CAD build for the part. Positions are in the model's coordinates, mm. Face numbers are marked on the shaded views. A direction names the side the tool comes from. Coordinates: 2 decimals unless noted, no trailing zeros. Order: outer loops, then holes, each group sorted by start corner. A loop starts at its lowest first (then second) coordinate and runs counter-clockwise, first axis right, second up. Notation, with made-up numbers: M -26,89 L -22,89 A21 cw -22,110 Z; hole C 58.5,19.5 d7. An arc over 180 degrees is marked long. Write item = value, one per line.
from build123d import *

# Parameters (mm, degrees)
F1_DEPTH = 60
F3_DEPTH = 2.001
F5_DEPTH = 1
F6_W     = 0.8
F6_H     = 3
F7_DEPTH = 1


# Not quite as in the source:
# - a feature names something its author has since deleted; it is built from what else it names


with BuildPart() as f1:
    # F0 (on Front) → F1 (new body)
    with BuildSketch(Plane.XZ):
        Polygon((0, 10), (0, 0), (16, 0), (16, 6), (13, 6.75), (13, 2), (3, 2), (3, 9.25), align=None)
    extrude(amount=F1_DEPTH)

    # F2 (on face) → F3 (cut, through all)
    with BuildSketch(Plane.XY.offset(2)):
        with BuildLine():
            ThreePointArc((12, -20.5), (8, -16.5), (4, -20.5))
            Line((4, -20.5), (4, -39.5))
            ThreePointArc((4, -39.5), (8, -43.5), (12, -39.5))
            Line((12, -39.5), (12, -20.5))
        make_face()
    extrude(amount=-F3_DEPTH, mode=Mode.SUBTRACT)

    # F4 (on Top) → F5 (cut)
    with BuildSketch(Plane.XY):
        with BuildLine():
            ThreePointArc((13, -20.5), (8, -15.5), (3, -20.5))
            Line((3, -20.5), (3, -39.5))
            ThreePointArc((3, -39.5), (8, -44.5), (13, -39.5))
            Line((13, -39.5), (13, -20.5))
        make_face()
    extrude(amount=F5_DEPTH, mode=Mode.SUBTRACT)

    # F6 (on Top) → F7 (join)
    with BuildSketch(Plane.XY):
        with Locations((6.8, -4.5)):
            Rectangle(F6_W, F6_H)
        with Locations((6.8, -55.5)):
            Rectangle(F6_W, F6_H)
    extrude(amount=-F7_DEPTH)


solid = f1.part
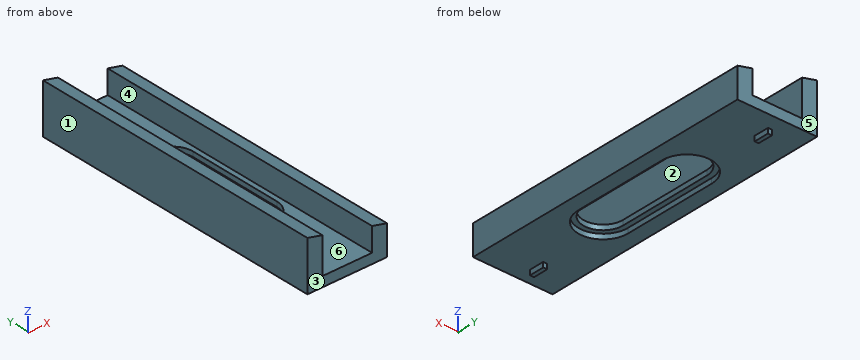
(1) Slice it at D-D, the plane y = -50. Write the cut outline in (x, z).
Evaluation:
outline = M 0,0 L 16,0 L 16,6 L 13,6.75 L 13,2 L 3,2 L 3,9.25 L 0,10 Z
(2) Pin check, flat tips, straight feed: pin 1 Ø5 at (x, y) = (6, -24.5) entering from -Z; pin 2 Ø5 at (x, y) = (12.5, -14) entering from +Z; pin 3 Ø0.5 at (y, z) = (-4.5, -0.5) entering from +X; pin 4 Ø3 at (x, y) = (9, -27) entering from -Z. Stop position of each tip, or through.
Evaluation:
pin_1 = 1
pin_2 = 6.75
pin_3 = 7.2
pin_4 = through
(3) Tool access for the marked faces 5 and 6: list every direction of +Z, -Z, +X, -X, +Y, -Y with a clear straight run to the whole face (end or side of a thin tool).
Evaluation:
face_5 = +Z, -Z, +X, -X, +Y
face_6 = +Z, +Y, -Y
(4) Pull direction X, two halves, no side cores. Call the marked faces 1, 2, 3 and 4: +X half, -X half, draft (parallel to the pull), parting line (faces both ways), or undercut.
Evaluation:
face_1 = -X half
face_2 = undercut
face_3 = draft
face_4 = undercut
(5) Slice it at C-C, the plane x = 8. Write the cut outline in (y, z).
Evaluation:
outline = M -60,0 L -44.5,0 L -44.5,1 L -43.5,1 L -43.5,2 L -60,2 Z; M -16.5,1 L -15.5,1 L -15.5,0 L 0,0 L 0,2 L -16.5,2 Z
(6) Slice it at A-A, the plane y = -31.5. Write the cut outline in (x, z), then the cut area to 3 significant figures.
Evaluation:
outline = M 0,0 L 3,0 L 3,1 L 4,1 L 4,2 L 3,2 L 3,9.25 L 0,10 Z; M 12,1 L 13,1 L 13,0 L 16,0 L 16,6 L 13,6.75 L 13,2 L 12,2 Z
area = 50.0 mm²
(7) Slice it at B-B, the plane z = 3. Write the cut outline in (x, y), then the cut area to 3 significant figures.
Evaluation:
outline = M 0,-60 L 3,-60 L 3,0 L 0,0 Z; M 13,-60 L 16,-60 L 16,0 L 13,0 Z
area = 360 mm²
(8) Wall check: line 1 (X direction, y = -34, z = 3.5); line 2 (Z direction, x = 6, y = -4); line 3 (X direction, y = -7, z = 7.75). Give the ranges that are in metal, low to high. Write a range as from..to.
Evaluation:
line_1 = 0..3, 13..16
line_2 = 0..2
line_3 = 0..3
